Source: CAD feature listing. Evaluate the final solid. Frame: model axes, mm. A direction names the side the tool comes from. Round coordinates to 2 decimals unless told otherwise and drop trailing zeros. Loops run counter-clockwise (first coordinate to the right, second up) from the corner with the lowest first, then second, coordinate; pieces in that order, holes last. Notation, with made-up numbers: (-30, 71) - (-10, 71) arc R20 ccw to (-10, 103) - close; hole circle Ø8 at (-28, -4.75). An arc over 180 degrees is marked (long way). One line per question, with ' | ' between items.
Autodesk Fusion 360 part; units mm, degrees
sketch "Sketch1" plane through (0, 0, 0) normal (0, 0, 1) x (1, 0, 0)
  line L0 (-17.3001, 65.9212) -> (152.6999, 65.9212)
  line L1 (152.6999, 65.9212) -> (152.6999, -74.0788)
  line L2 (152.6999, -74.0788) -> (-17.3001, -74.0788)
  line L3 (-17.3001, -74.0788) -> (-17.3001, 65.9212)
  dimension "d1" = 140
  dimension "d2" = 170
extrude "Extrude1" add sketch "Sketch1" along normal blind 5
sketch "Sketch10" plane through (0, 0, 5) normal (0, 0, 1) x (-1, 0, 0)
  line L0 (17.3001, 74.0788) -> (-152.6999, 74.0788)
  line L1 (-152.6999, 74.0788) -> (-152.6999, -65.9212)
  line L2 (-152.6999, -65.9212) -> (17.3001, -65.9212)
  line L3 (17.3001, -65.9212) -> (17.3001, 74.0788)
  line L4 (-7.6999, -40.9212) -> (-127.6999, -40.9212)
  line L5 (-127.6999, -40.9212) -> (-127.6999, 49.0788)
  line L6 (-127.6999, 49.0788) -> (-7.6999, 49.0788)
  line L7 (-7.6999, 49.0788) -> (-7.6999, -40.9212)
  line L8 (17.3001, -65.9212) -> (-152.6999, -65.9212)
  line L9 (-152.6999, 74.0788) -> (17.3001, 74.0788)
  line L10 (17.3001, 74.0788) -> (17.3001, -65.9212)
  line L11 (-152.6999, -65.9212) -> (-152.6999, 74.0788)
  line L12 (-2.5999, -46.0212) -> (-12.7999, -46.0212)
  line L13 (-12.7999, -46.0212) -> (-12.7999, -35.8212)
  line L14 (-12.7999, -35.8212) -> (-2.5999, -35.8212)
  line L15 (-2.5999, -35.8212) -> (-2.5999, -46.0212)
  line L16 (-122.5999, -46.0212) -> (-132.7999, -46.0212)
  line L17 (-132.7999, -46.0212) -> (-132.7999, -35.8212)
  line L18 (-132.7999, -35.8212) -> (-122.5999, -35.8212)
  line L19 (-122.5999, -35.8212) -> (-122.5999, -46.0212)
  line L20 (-62.5999, -46.0212) -> (-72.7999, -46.0212)
  line L21 (-72.7999, -46.0212) -> (-72.7999, -35.8212)
  line L22 (-72.7999, -35.8212) -> (-62.5999, -35.8212)
  line L23 (-62.5999, -35.8212) -> (-62.5999, -46.0212)
  line L24 (-2.5999, 43.9788) -> (-12.7999, 43.9788)
  line L25 (-12.7999, 43.9788) -> (-12.7999, 54.1788)
  line L26 (-12.7999, 54.1788) -> (-2.5999, 54.1788)
  line L27 (-2.5999, 54.1788) -> (-2.5999, 43.9788)
  line L28 (-122.5999, 43.9788) -> (-132.7999, 43.9788)
  line L29 (-132.7999, 43.9788) -> (-132.7999, 54.1788)
  line L30 (-132.7999, 54.1788) -> (-122.5999, 54.1788)
  line L31 (-122.5999, 54.1788) -> (-122.5999, 43.9788)
  line L32 (-62.5999, 43.9788) -> (-72.7999, 43.9788)
  line L33 (-72.7999, 43.9788) -> (-72.7999, 54.1788)
  line L34 (-72.7999, 54.1788) -> (-62.5999, 54.1788)
  line L35 (-62.5999, 54.1788) -> (-62.5999, 43.9788)
  line L36 (-22.6999, -25.9212) -> (-112.6999, -25.9212)
  line L37 (-112.6999, -25.9212) -> (-112.6999, 34.0788)
  line L38 (-112.6999, 34.0788) -> (-22.6999, 34.0788)
  line L39 (-22.6999, 34.0788) -> (-22.6999, -25.9212)
  line L40 (2.4001, -51.0212) -> (-17.7999, -51.0212)
  line L41 (-17.7999, -51.0212) -> (-17.7999, -30.8212)
  line L42 (-17.7999, -30.8212) -> (2.4001, -30.8212)
  line L43 (2.4001, -30.8212) -> (2.4001, -51.0212)
  line L44 (-57.5999, -51.0212) -> (-77.7999, -51.0212)
  line L45 (-77.7999, -51.0212) -> (-77.7999, -30.8212)
  line L46 (-77.7999, -30.8212) -> (-57.5999, -30.8212)
  line L47 (-57.5999, -30.8212) -> (-57.5999, -51.0212)
  line L48 (-117.5999, -51.0212) -> (-137.7999, -51.0212)
  line L49 (-137.7999, -51.0212) -> (-137.7999, -30.8212)
  line L50 (-137.7999, -30.8212) -> (-117.5999, -30.8212)
  line L51 (-117.5999, -30.8212) -> (-117.5999, -51.0212)
  line L52 (-117.5999, 38.9788) -> (-137.7999, 38.9788)
  line L53 (-137.7999, 38.9788) -> (-137.7999, 59.1788)
  line L54 (-137.7999, 59.1788) -> (-117.5999, 59.1788)
  line L55 (-117.5999, 59.1788) -> (-117.5999, 38.9788)
  line L56 (-57.5999, 38.9788) -> (-77.7999, 38.9788)
  line L57 (-77.7999, 38.9788) -> (-77.7999, 59.1788)
  line L58 (-77.7999, 59.1788) -> (-57.5999, 59.1788)
  line L59 (-57.5999, 59.1788) -> (-57.5999, 38.9788)
  line L60 (2.4001, 38.9788) -> (-17.7999, 38.9788)
  line L61 (-17.7999, 38.9788) -> (-17.7999, 59.1788)
  line L62 (-17.7999, 59.1788) -> (2.4001, 59.1788)
  line L63 (2.4001, 59.1788) -> (2.4001, 38.9788)
  dimension "d65" = 25
  dimension "d66" = 25
  dimension "d67" = 25
  dimension "d68" = 25
  dimension "d69" = 5.1
  dimension "d70" = 5.1
  dimension "d71" = 5.1
  dimension "d72" = 5.1
  dimension "d73" = 5.1
  dimension "d74" = 5.1
  dimension "d75" = 5.1
  dimension "d76" = 5.1
  dimension "d77" = 109.8
  dimension "d78" = 19.9
  dimension "d79" = 19.9
  dimension "d80" = 49.8
  dimension "d81" = 49.8
  dimension "d82" = 5.1
  dimension "d83" = 5.1
  dimension "d84" = 5.1
  dimension "d85" = 5.1
  dimension "d86" = 5.1
  dimension "d87" = 5.1
  dimension "d88" = 5.1
  dimension "d89" = 5.1
  dimension "d90" = 5.1
  dimension "d91" = 5.1
  dimension "d92" = 49.8
  dimension "d93" = 49.8
  dimension "d94" = 5.1
  dimension "d95" = 5.1
  dimension "d96" = 15
  dimension "d97" = 15
  dimension "d98" = 15
  dimension "d99" = 15
  dimension "d100" = 5
  dimension "d101" = 5
  dimension "d102" = 5
  dimension "d103" = 5
  dimension "d104" = 5
  dimension "d105" = 5
  dimension "d106" = 5
  dimension "d107" = 5
  dimension "d108" = 5
  dimension "d109" = 5
  dimension "d110" = 5
  dimension "d111" = 5
  dimension "d112" = 5
  dimension "d113" = 5
  dimension "d114" = 5
  dimension "d115" = 5
  dimension "d116" = 5
  dimension "d117" = 5
  dimension "d118" = 5
  dimension "d119" = 5
  dimension "d120" = 5
  dimension "d121" = 5
  dimension "d122" = 5
  dimension "d123" = 5
extrude "Extrude8" cut sketch "Sketch10" against normal blind 5 contours L36 L37 L38 L39
extrude "Extrude9" cut sketch "Sketch10" against normal blind 2.5 contours L4 L7 L12 L13 L14 L15 | L4 L7 L13 L14 | L4 L20 L21 L23 | L4 L21 L22 L23 | L6 L7 L24 L25 | L6 L7 L24 L25 L26 L27 | L6 L32 L33 L35 | L6 L33 L34 L35 | L4 L5 L16 L17 L18 L19 | L4 L5 L18 L19 | L5 L6 L28 L29 L30 L31 | L5 L6 L28 L31
extrude "Extrude10" add sketch "Sketch10" along normal blind 10 contours L4 L7 L12 L13 L14 L15 L40 L41 L42 L43 | L4 L7 L13 L14 L41 L42 | L4 L20 L21 L23 L44 L45 L47 | L4 L21 L22 L23 L45 L46 L47 | L6 L7 L24 L25 L60 L61 | L6 L7 L24 L25 L26 L27 L60 L61 L62 L63 | L6 L32 L33 L35 L56 L57 L59 | L6 L33 L34 L35 L57 L58 L59 | L4 L5 L16 L17 L18 L19 L48 L49 L50 L51 | L4 L5 L18 L19 L50 L51 | L5 L6 L28 L29 L30 L31 L52 L53 L54 L55 | L5 L6 L28 L31 L52 L55
fillet "Fillet1" radius 2 4 edges at (152.6999, -74.0788, 2.5) (152.6999, 65.9212, 2.5) (-17.3001, 65.9212, 2.5) (-17.3001, -74.0788, 2.5)
extrude "Extrude11" add 6 faces at (5.9999, 49.3545, 15) (76.1332, 39.2212, 15) (136.1332, 39.2212, 15) (136.1332, -50.7788, 15) (76.1332, -50.7788, 15) (5.9999, -40.6455, 15) along direction (0, 0, 1) blind 10
fillet "Fillet2" radius 2 24 edges at (17.7999, 30.8212, 15) (-2.4001, 30.8212, 15) (57.5999, 30.8212, 15) (77.7999, 30.8212, 15) (117.5999, 30.8212, 15) (137.7999, 30.8212, 15) (57.5999, -59.1788, 15) (77.7999, -59.1788, 15) (17.7999, -59.1788, 15) (-2.4001, -59.1788, 15) (-2.4001, -38.9788, 15) (-2.4001, 51.0212, 15) (57.5999, 51.0212, 15) (117.5999, 51.0212, 15) (117.5999, -38.9788, 15) (117.5999, -59.1788, 15) (57.5999, -38.9788, 15) (77.7999, -38.9788, 15) (137.7999, -59.1788, 15) (137.7999, -38.9788, 15) (77.7999, 51.0212, 15) (137.7999, 51.0212, 15) (17.7999, 51.0212, 15) (17.7999, -38.9788, 15)
fillet "Fillet3" radius 2 4 edges at (22.6999, 25.9212, 2.5) (22.6999, -34.0788, 2.5) (112.6999, -34.0788, 2.5) (112.6999, 25.9212, 2.5)
1. Section query A-A, the plane y = -16.5. Return loops of the section in (x, z).
Worked out:
outline: (-17.3, 0) - (22.7, 0) - (22.7, 5) - (-17.3, 5) - close; (112.7, 0) - (152.7, 0) - (152.7, 5) - (112.7, 5) - close
2. Contact query for flat-ended pins moving along their axis: P1, Ø8, axis at x = 6, z = 10.5, coming from the +Y side; P2, Ø3, axis at y = -55.5, z = 20.5, coming from the +X side; P3, Ø8, axis at x = 8, z = 14.5, coming from the -Y side. Output: stop coordinate, or through.
Worked out:
P1: stops at y = 51.02 | P2: stops at x = 137.8 | P3: stops at y = -59.18
3. Mould query, pull axis X, two halves, no side actions, for faces 5 (the flat face through (152.7, -3, 2)), 6 (the flat face through (67, 28, 0)), 7 (the flat face through (8, 35.821, 14)). Classes: released by +X, released by -X, zero draft, split by the parting line, or undercut.
Worked out:
face 5: released by +X | face 6: zero draft | face 7: undercut
4. Access query for faces 1 (the flat face through (128, -49, 2.5)), 2 (the flat face through (77.8, 41, 15)), 3 (the flat face through (22.7, -4, 3)), 4 (the flat face through (8, -59.179, 15)). Directions: +Z, -Z, +X, -X, +Y, -Y. A direction counts if a zero-diameter tool reaches every point of the face in a straight line with its end or side. Return the directions, or none.
Worked out:
face 1: +Z | face 2: +Z, +Y, -Y | face 3: +Z, -Z | face 4: +Z, +X, -X, -Y
5. Section query D-D, the plane z = 19.75. Give the number of separate pieces and of enclosed holes in the cut face, plus the area to 3 significant figures.
Worked out:
separate pieces: 6 | enclosed holes: 6 | area: 1,800 mm2
6. Material intervals for probe 1 along X at (y, z) = (-54.5, 5.5); probe 2 along Y at (x, z) = (123, 20.25); probe 3 along X at (y, z) = (43.5, 8.5), sorted ascending.
Worked out:
probe 1: x = -2.4 to 17.8, 57.6 to 77.8, 117.6 to 137.8 | probe 2: y = -59.18 to -54.18, -43.98 to -38.98, 30.82 to 35.82, 46.02 to 51.02 | probe 3: x = -2.4 to 2.6, 12.8 to 17.8, 57.6 to 62.6, 72.8 to 77.8, 117.6 to 122.6, 132.8 to 137.8
7. Section query B-B, the plane x = 88.5. Return loops of the section in (y, z).
Worked out:
outline: (-74.08, 0) - (-34.08, 0) - (-34.08, 5) - (-74.08, 5) - close; (25.92, 0) - (65.92, 0) - (65.92, 5) - (25.92, 5) - close
8. Section query C-C, the plane x = 129. Return loops of the section in (y, z), plus the area to 3 significant figures.
Worked out:
outline: (-74.08, 0) - (65.92, 0) - (65.92, 5) - (51.02, 5) - (51.02, 25) - (46.02, 25) - (46.02, 2.5) - (35.82, 2.5) - (35.82, 25) - (30.82, 25) - (30.82, 5) - (-38.98, 5) - (-38.98, 25) - (-43.98, 25) - (-43.98, 2.5) - (-54.18, 2.5) - (-54.18, 25) - (-59.18, 25) - (-59.18, 5) - (-74.08, 5) - close | area: 1,050 mm2
